Can you work these out from the model? Positions are in its coordinate system, mm. Coordinates: 2 decimals unless noted, no trailing zeros. Loops run counter-clockwise (first coordinate to the right, second up) from the corner with the lowest first, then second, coordinate; pieces in that order, holes last. Notation, with made-up numbers: (9.25, 28.5) -> (48.25, 28.5) arc R10 cw to (48.25, 38.5) -> close; hole circle Ø3 at (-0.75, -8.5). An arc over 180 degrees is marked (long way). Use one line per item in the form item = value. Start each with the question number.
(1) I'm going to push flat-ended pins straight in: pin 1 (1.5 mm diameter, centred on y = -0.5, z = 7.5, fed in from +X); pin 2 (10 mm diameter, centred on x = -8, z = 1.5, fed in from +Y). Where does each tip first touch, or does it pass through?
(2) Imagine slicing it at C-C (x = -8). List the corners of the cut face in (y, z) for me.
(3) Imagine slicing it at A-A (z = 0). List the corners of the cut face in (x, y) for me.
(4) Imagine slicing it at B-B (x = 0). List the corners of the cut face in (y, z) for me (3 decimals).
(5) Imagine slicing it at D-D (x = -15.5). List the corners of the cut face in (y, z) for me, plus the area to 3 significant figures.
(6) I need wall thicknesses on line 1 (Z direction, x = 0, y = -2.4) (3 decimals); line 2 (Z direction, x = 2.5, y = -1.4); line 3 (Z direction, x = -15.5, y = -2.2). Which ranges of each line are inside material? Lowest first, please. Write a range as [from, to].
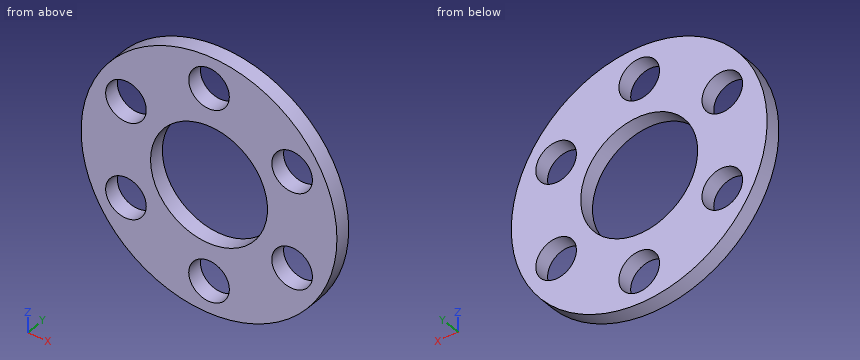
```python
from build123d import *

# Parameters (mm, degrees)
F0_R            = 20
F1_DEPTH        = 2.54
F2_R            = 9.144
F3_DEPTH        = 8.5
F4_R            = 3.175
F5_DEPTH        = 2.541
F5_COPIES_COUNT = 6


# Not quite as in the source:
# - a pattern or mirror of a feature is missing from the dataset's text; its kind, count and spacing are read off the source's solid


with BuildPart() as f1:
    # F0 (on Front) → F1 (new body)
    with BuildSketch(Plane.XZ):
        Circle(F0_R)
    extrude(amount=F1_DEPTH)

    # F2 (on face) → F3 (cut)
    with BuildSketch(Plane(origin=(0, 0, 0), x_dir=(-1, 0, 0), z_dir=(0, 1, 0))):
        Circle(F2_R)
    extrude(amount=-F3_DEPTH, mode=Mode.SUBTRACT)

    # F4 (on face) → F5 (cut, through all)
    with BuildSketch(Plane.XZ.offset(2.54)):
        with Locations((0, 15)):
            Circle(F4_R)
    f5 = extrude(amount=-F5_DEPTH, mode=Mode.SUBTRACT)

    # F5_copies: F5 ×6 about axis
    f5_copies_axis = Axis((0, 0, 0), (0, 1, 0))
    for i in range(1, F5_COPIES_COUNT):
        add(f5.rotate(f5_copies_axis, i * 360 / F5_COPIES_COUNT), mode=Mode.SUBTRACT)


solid = f1.part
```
Worked out:
q1.pin_1 = 18.83
q1.pin_2 = 0
q2.outline = (-2.54, -18.33) -> (0, -18.33) -> (0, -4.43) -> (-2.54, -4.43) -> close; (-2.54, 4.43) -> (0, 4.43) -> (0, 18.33) -> (-2.54, 18.33) -> close
q3.outline = (-20, -2.54) -> (-9.14, -2.54) -> (-9.14, 0) -> (-20, 0) -> close; (9.14, -2.54) -> (20, -2.54) -> (20, 0) -> (9.14, 0) -> close
q4.outline = (-2.54, -20) -> (0, -20) -> (0, -18.175) -> (-2.54, -18.175) -> close; (-2.54, -11.825) -> (0, -11.825) -> (0, -9.144) -> (-2.54, -9.144) -> close; (-2.54, 9.144) -> (0, 9.144) -> (0, 11.825) -> (-2.54, 11.825) -> close; (-2.54, 18.175) -> (0, 18.175) -> (0, 20) -> (-2.54, 20) -> close
q5.outline = (-2.54, -12.64) -> (0, -12.64) -> (0, -9.44) -> (-2.54, -9.44) -> close; (-2.54, -5.56) -> (0, -5.56) -> (0, 5.56) -> (-2.54, 5.56) -> close; (-2.54, 9.44) -> (0, 9.44) -> (0, 12.64) -> (-2.54, 12.64) -> close
q5.area = 44.4 mm2
q6.line_1 = [-20, -18.175], [-11.825, -9.144], [9.144, 11.825], [18.175, 20]
q6.line_2 = [-19.84, -16.96], [-13.04, -8.8], [8.8, 13.04], [16.96, 19.84]
q6.line_3 = [-12.64, -9.44], [-5.56, 5.56], [9.44, 12.64]
